Read the model definition and answer for the solid it produces. Units are mm, in the model's axes. Give positions to 0.01 mm unless a question says otherwise; leave off trailing zeros. Write each loop counter-clockwise with the first axis right and the second up, starting at its lowest first coordinate (ties: lowest second). Pieces come first, ordered by that corner, then holes. Notation, with made-up numbers: (68.5, 86) - (93.5, 86) arc R26 cw to (93.5, 107) - close; hole circle Ø7 at (3.5, 19). An arc over 180 degrees is marked (long way). Answer as CSV lines item,"result".
```python
from build123d import *

# Parameters (mm, degrees)
SKETCH1_W           = 120
SKETCH1_H           = 80
SKETCH1_R           = 1.6
SKETCH1_R_2         = 11.25
BOSS_EXTRUDE3_DEPTH = 4
FILLET5_R           = 2
FILLET6_R           = 2
FILLET7_R           = 2
FILLET8_R           = 2


with BuildPart() as part:
    # Sketch1 → Boss-Extrude3 (new body)
    with BuildSketch(Plane(origin=(0, 0, 0), x_dir=(1, 0, 0), z_dir=(0, 1, 0))):
        with Locations((60, 40)):
            Rectangle(SKETCH1_W, SKETCH1_H)
        with Locations((3, 77)):
            Circle(SKETCH1_R, mode=Mode.SUBTRACT)
        with Locations((3, 3)):
            Circle(SKETCH1_R, mode=Mode.SUBTRACT)
        with Locations((117, 77)):
            Circle(SKETCH1_R, mode=Mode.SUBTRACT)
        with Locations((117, 3)):
            Circle(SKETCH1_R, mode=Mode.SUBTRACT)
        with Locations((110, 59)):
            Circle(SKETCH1_R, mode=Mode.SUBTRACT)
        with Locations((94.8, 8.2)):
            Circle(SKETCH1_R, mode=Mode.SUBTRACT)
        with Locations((66.9, 8.2)):
            Circle(SKETCH1_R, mode=Mode.SUBTRACT)
        with Locations((11.9, 8.2)):
            Circle(SKETCH1_R, mode=Mode.SUBTRACT)
        with Locations((48.9, 8.2)):
            Circle(SKETCH1_R, mode=Mode.SUBTRACT)
        with Locations((11.9, 45.2)):
            Circle(SKETCH1_R, mode=Mode.SUBTRACT)
        with Locations((48.9, 45.2)):
            Circle(SKETCH1_R, mode=Mode.SUBTRACT)
        with Locations((11.9, 55.2)):
            Circle(SKETCH1_R, mode=Mode.SUBTRACT)
        with Locations((27.9, 55.2)):
            Circle(SKETCH1_R, mode=Mode.SUBTRACT)
        with Locations((45, 62)):
            Circle(SKETCH1_R_2, mode=Mode.SUBTRACT)
        with Locations((62.2, 60.1)):
            Circle(SKETCH1_R, mode=Mode.SUBTRACT)
        with BuildLine():
            Line((10, 77.75), (110, 77.75))
            ThreePointArc((110, 77.75), (110.75, 77), (110, 76.25))
            Line((110, 76.25), (10, 76.25))
            ThreePointArc((10, 76.25), (9.25, 77), (10, 77.75))
        make_face(mode=Mode.SUBTRACT)
        with BuildLine():
            Line((3.75, 70), (3.75, 10))
            ThreePointArc((3.75, 10), (3, 9.25), (2.25, 10))
            Line((2.25, 10), (2.25, 70))
            ThreePointArc((2.25, 70), (3, 70.75), (3.75, 70))
        make_face(mode=Mode.SUBTRACT)
        with BuildLine():
            Line((10, 3.75), (110, 3.75))
            ThreePointArc((110, 3.75), (110.75, 3), (110, 2.25))
            Line((110, 2.25), (10, 2.25))
            ThreePointArc((10, 2.25), (9.25, 3), (10, 3.75))
        make_face(mode=Mode.SUBTRACT)
        with BuildLine():
            Line((117.75, 70), (117.75, 10))
            ThreePointArc((117.75, 10), (117, 9.25), (116.25, 10))
            Line((116.25, 10), (116.25, 70))
            ThreePointArc((116.25, 70), (117, 70.75), (117.75, 70))
        make_face(mode=Mode.SUBTRACT)
    extrude(amount=BOSS_EXTRUDE3_DEPTH)

    # Fillet5
    fillet5_edges = [part.edges().sort_by_distance(p)[0] for p in [
        (0, 2, 0),
    ]]
    fillet(fillet5_edges, radius=FILLET5_R)

    # Fillet6
    fillet6_edges = [part.edges().sort_by_distance(p)[0] for p in [
        (0, 2, -80),
    ]]
    fillet(fillet6_edges, radius=FILLET6_R)

    # Fillet7
    fillet7_edges = [part.edges().sort_by_distance(p)[0] for p in [
        (120, 2, -80),
    ]]
    fillet(fillet7_edges, radius=FILLET7_R)

    # Fillet8
    fillet8_edges = [part.edges().sort_by_distance(p)[0] for p in [
        (120, 2, 0),
    ]]
    fillet(fillet8_edges, radius=FILLET8_R)


solid = part.part
```
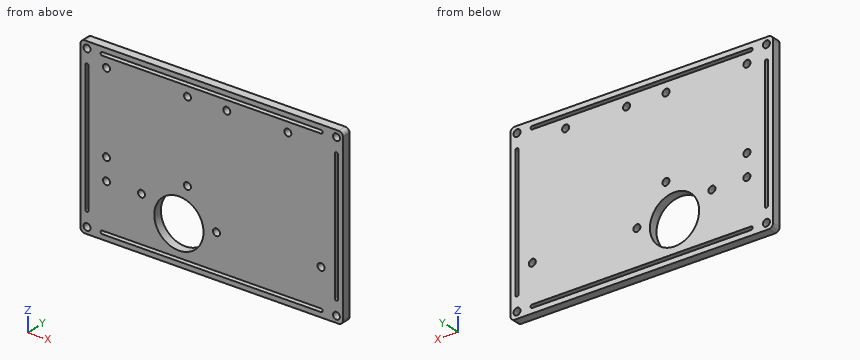
(1) A cutting plane is placed at C-C (x = 62.2). Write down the section's boundary in (y, z), and give its area (3 significant figures).
Worked out:
outline,"(0, -80) - (4, -80) - (4, -77.75) - (0, -77.75) - close; (0, -76.25) - (4, -76.25) - (4, -61.7) - (0, -61.7) - close; (0, -58.5) - (4, -58.5) - (4, -3.75) - (0, -3.75) - close; (0, -2.25) - (4, -2.25) - (4, 0) - (0, 0) - close"
area,"295 mm^2"
(2) Find the intervals of material crossed by L1, parallel to X at y = 3.2, z = -39; L2, parallel to Z at x = 62, y = 2.25; L3, parallel to Z at x = 14, y = 1, in increasing order.
Worked out:
L1,"x = 0 to 2.25, 3.75 to 116.25, 117.75 to 120"
L2,"z = -80 to -77.75, -76.25 to -61.69, -58.51 to -3.75, -2.25 to 0"
L3,"z = -80 to -77.75, -76.25 to -3.75, -2.25 to 0"
(3) A cutting plane is placed at B-B (z = -45.2). Write down the section's boundary in (x, y).
Worked out:
outline,"(0, 0) - (2.25, 0) - (2.25, 4) - (0, 4) - close; (3.75, 0) - (10.3, 0) - (10.3, 4) - (3.75, 4) - close; (13.5, 0) - (47.3, 0) - (47.3, 4) - (13.5, 4) - close; (50.5, 0) - (116.25, 0) - (116.25, 4) - (50.5, 4) - close; (117.75, 0) - (120, 0) - (120, 4) - (117.75, 4) - close"
(4) A cutting plane is placed at A-A (x = 15). Write down the section's boundary in (y, z), and give its area (3 significant figures).
Worked out:
outline,"(0, -80) - (4, -80) - (4, -77.75) - (0, -77.75) - close; (0, -76.25) - (4, -76.25) - (4, -3.75) - (0, -3.75) - close; (0, -2.25) - (4, -2.25) - (4, 0) - (0, 0) - close"
area,"308 mm^2"
(5) A cutting plane is placed at D-D (z = -18). Write down the section's boundary in (x, y).
Worked out:
outline,"(0, 0) - (2.25, 0) - (2.25, 4) - (0, 4) - close; (3.75, 0) - (116.25, 0) - (116.25, 4) - (3.75, 4) - close; (117.75, 0) - (120, 0) - (120, 4) - (117.75, 4) - close"
